from build123d import *

# Parameters (mm, degrees)
F1_DEPTH = 76.2
F3_DEPTH = 76.2
F5_DEPTH = 152.4


with BuildPart() as f1:
    # F0 (on Front) → F1 (new body)
    with BuildSketch(Plane.XZ):
        Polygon((0, 50.8), (0, 0), (152.4, 0), (152.4, 38.1), (85.151714, 38.1), (76.2, 50.8), align=None)
    extrude(amount=-F1_DEPTH)

    # F2 (on face) → F3 (cut)
    with BuildSketch(Plane.XZ):
        Polygon((56.892031, 50.8), (31.492031, 50.8), (31.492031, 38.1), (18.792031, 38.1), (18.792031, 25.4), (69.592031, 25.4), (69.592031, 38.1), (56.892031, 38.1), align=None)
    extrude(amount=-F3_DEPTH, mode=Mode.SUBTRACT)

    # F4 (on face) → F5 (cut)
    with BuildSketch(Plane.YZ.offset(152.4)):
        Polygon((63.962197, 17.182477), (13.162197, 17.182477), (25.314642, 0), (50.714642, 0), align=None)
    extrude(amount=-F5_DEPTH, mode=Mode.SUBTRACT)


solid = f1.part
Work out the finished part from the listing and answer in its coordinate system (mm). A direction names the side the tool comes from. Give positions to 0.01 mm unless a question says otherwise; leave off trailing zeros. Write each loop counter-clockwise with the first axis right and the second up, starting at its lowest first coordinate (ties: lowest second). Pieces come first, ordered by that corner, then holes.
Q1. Straight lines are drawn through the part: L1, parallel to Z at x = 65, y = 35.5; L2, parallel to Z at x = 62, y = 11; L3, parallel to X at y = 68.5, z = 35. For each, find the intervals that lie inside material, in ascending order.
Answer:
L1: z = 17.18 to 25.4, 38.1 to 50.8
L2: z = 0 to 25.4, 38.1 to 50.8
L3: x = 0 to 18.79, 69.59 to 152.4
Q2. Given pin 1 (3 mm diameter, centred on x = 51, y = 8, fed in from +Z); pin 2 (20 mm diameter, centred on x = 121, y = 36, fed in from +Z); pin 3 (6.5 mm diameter, centred on x = 26, y = 29, fed in from -Z), each flat-ended and moving along its own axis, determine where each tip first touches the part or whether it passes through.
Answer:
pin 1: stops at z = 25.4
pin 2: stops at z = 38.1
pin 3: stops at z = 17.18
Q3. The part is cut by section B-B on y = 56.5. Give the vertices of the cut face in (x, z), and give its area (3 significant figures).
Answer:
outline: (0, 0) - (152.4, 0) - (152.4, 7.5) - (0, 7.5) - close; (0, 17.18) - (152.4, 17.18) - (152.4, 38.1) - (85.15, 38.1) - (76.2, 50.8) - (56.89, 50.8) - (56.89, 38.1) - (69.59, 38.1) - (69.59, 25.4) - (18.79, 25.4) - (18.79, 38.1) - (31.49, 38.1) - (31.49, 50.8) - (0, 50.8) - close
area: 4,390 mm2
Q4. For a pull along X with two mould halves and no side action, classify faces 6 (the face through (152.4, 38, 23)), 7 (the face through (75, 0, 20)), 8 (the face through (63, 38, 38.1)) as released by +X, released by -X, zero draft, split by the parting line, or undercut.
Answer:
face 6: released by +X
face 7: zero draft
face 8: undercut
Q5. The part is cut by section D-D on y = 41.5. Give the vertices of the cut face in (x, z).
Answer:
outline: (0, 17.18) - (152.4, 17.18) - (152.4, 38.1) - (85.15, 38.1) - (76.2, 50.8) - (56.89, 50.8) - (56.89, 38.1) - (69.59, 38.1) - (69.59, 25.4) - (18.79, 25.4) - (18.79, 38.1) - (31.49, 38.1) - (31.49, 50.8) - (0, 50.8) - close
Q6. The part is cut by section A-A on z = 35.5. Give the vertices of the cut face in (x, y).
Answer:
outline: (0, 0) - (18.79, 0) - (18.79, 76.2) - (0, 76.2) - close; (69.59, 0) - (152.4, 0) - (152.4, 76.2) - (69.59, 76.2) - close
Q7. A tool of negligible diameter and unlimited length cuts with its end or side. For faces 1 (the face through (75, 63, 0)), 2 (the face through (77, 39, 17.182)), 3 (the face through (56.892, 38, 44)), 4 (the face through (44, 38, 25.4)), 5 (the face through (119, 38, 38.1)), from which of +Z, -Z, +X, -X, +Y, -Y can it reach the whole face along a straight path? Write none if from no direction.
Answer:
face 1: -Z, +X, -X, +Y, -Y
face 2: +X, -X
face 3: +Z, +Y, -Y
face 4: +Y, -Y
face 5: +Z, +X, +Y, -Y
Q8. The part is cut by section C-C on x = 74. Give the vertices of the cut face in (y, z), and give its area (3 significant figures).
Answer:
outline: (0, 0) - (25.31, 0) - (13.16, 17.18) - (63.96, 17.18) - (50.71, 0) - (76.2, 0) - (76.2, 50.8) - (0, 50.8) - close
area: 3,220 mm2
